```python
from build123d import *

# Parameters (mm, degrees)
SKETCH_1_R          = 1.75
EXTRUDE_1_DEPTH     = 5
CUT_EXTRUDE_1_REACH = 7
SKETCH_2_W          = 35
SKETCH_2_H          = 3


with BuildPart() as part:
    # 草圖1 → 填料-伸長1 (new body)
    with BuildSketch(Plane.XY):
        Polygon((-30, 28.5), (-30, 20.5), (-22, 20.5), (-22, -20.5), (-30, -20.5), (-30, -28.5), (30, -28.5), (30, -20.5), (22, -20.5), (22, 20.5), (30, 20.5), (30, 28.5), align=None)
        with Locations((-26, 24.5)):
            Circle(SKETCH_1_R, mode=Mode.SUBTRACT)
        with Locations((26, 24.5)):
            Circle(SKETCH_1_R, mode=Mode.SUBTRACT)
        with Locations((-26, -24.5)):
            Circle(SKETCH_1_R, mode=Mode.SUBTRACT)
        with Locations((26, -24.5)):
            Circle(SKETCH_1_R, mode=Mode.SUBTRACT)
    extrude(amount=EXTRUDE_1_DEPTH)

    # 草圖2 → 除料-伸長1 (cut, up to next)
    with BuildSketch(Plane.XY.offset(5), mode=Mode.PRIVATE) as cut_extrude_1_sk1:
        with Locations((0, -19)):
            Rectangle(SKETCH_2_W, SKETCH_2_H)
    cut_extrude_1_tool1 = extrude(cut_extrude_1_sk1.sketch, amount=-CUT_EXTRUDE_1_REACH, mode=Mode.PRIVATE) & part.part
    add(cut_extrude_1_tool1.solids().sort_by_distance((0, -19, 5))[0], mode=Mode.SUBTRACT)


solid = part.part
```
Part model, mm, in its own coordinate system. A direction names the side the tool comes from. Round coordinates to 2 decimals unless told otherwise and drop trailing zeros. Order: outer loops, then holes, each group sorted by start corner. A loop starts at its lowest first (then second) coordinate and runs counter-clockwise, first axis right, second up. Notation, with made-up numbers: M 73.5,-9 L 125.5,-9 A21 cw 125.5,12 Z; hole C -27,8.25 d3. An arc over 180 degrees is marked long. Put each result on its own line as item: value. Start each with the question number.
1. Slice it at A-A on x = 26. List the corners of the cut face in (y, z), then the cut area to 3 significant figures.
2. Tool access for faces 1 (the face through (-26, -20.5, 2)), 2 (the face through (30, -25, 2)), 3 (the face through (-17.5, -19, 3)), 4 (the face through (22, 0, 2)): list every direction of +Z, -Z, +X, -X, +Y, -Y with a clear straight run to the whole face (end or side of a thin tool).
3. Slice it at D-D on z = 2.3. List the corners of the cut face in (x, y).
4. Two-plate mould, pull along Y, no slides. Class faces 5 (the face through (26, 20.5, 2)), 6 (the face through (0, -17.5, 3)), 7 (the face through (0, -28.5, 2)), 8 (the face through (-30, 25, 2)): +Y half, -Y half, draft (parallel to the pull), parting line (faces both ways), or undercut.
5. Slice it at B-B on y = -24.5. List the corners of the cut face in (x, z), then the cut area to 3 significant figures.
6. Drill centre lines: probe 1 along Y at (x, z) = (26, 2.7); probe 2 along Y at (x, z) = (22.5, 0.35); probe 3 along Y at (x, z) = (-12.5, 1.15). Where is each one in solid material? Low to high. Write a range as [from, to].
7. Slice it at C-C on x = 3. List the corners of the cut face in (y, z).
8. Drop flat-ended pins along their axis: pin 1 (3 mm diameter, centred on x = -26, y = -24.5, fed in from -Z); pin 2 (3 mm diameter, centred on y = 9, z = 3.5, fed in from +X). Give the stop position or say it passes through.
Findings:
1. outline: M -28.5,0 L -26.25,0 L -26.25,5 L -28.5,5 Z; M -22.75,0 L -20.5,0 L -20.5,5 L -22.75,5 Z; M 20.5,0 L 22.75,0 L 22.75,5 L 20.5,5 Z; M 26.25,0 L 28.5,0 L 28.5,5 L 26.25,5 Z
1. area: 45.0 mm2
2. face 1: +Z, -Z, -X
2. face 2: +Z, -Z, +X, +Y, -Y
2. face 3: +Z, -Z
2. face 4: +Z, -Z, +X
3. outline: M -30,-28.5 L 30,-28.5 L 30,-20.5 L 22,-20.5 L 22,20.5 L 30,20.5 L 30,28.5 L -30,28.5 L -30,20.5 L -22,20.5 L -22,-20.5 L -30,-20.5 Z; hole C -26,-24.5 d3.5; hole C -26,24.5 d3.5; hole M -17.5,-20.5 L 17.5,-20.5 L 17.5,-17.5 L -17.5,-17.5 Z; hole C 26,-24.5 d3.5; hole C 26,24.5 d3.5
4. face 5: undercut
4. face 6: undercut
4. face 7: -Y half
4. face 8: draft
5. outline: M -30,0 L -27.75,0 L -27.75,5 L -30,5 Z; M -24.25,0 L 24.25,0 L 24.25,5 L -24.25,5 Z; M 27.75,0 L 30,0 L 30,5 L 27.75,5 Z
5. area: 265 mm2
6. probe 1: [-28.5, -26.25], [-22.75, -20.5], [20.5, 22.75], [26.25, 28.5]
6. probe 2: [-28.5, -20.5], [20.5, 28.5]
6. probe 3: [-28.5, -20.5], [-17.5, 28.5]
7. outline: M -28.5,0 L -20.5,0 L -20.5,5 L -28.5,5 Z; M -17.5,0 L 28.5,0 L 28.5,5 L -17.5,5 Z
8. pin 1: through
8. pin 2: x = 22
